from build123d import *

# Parameters (mm, degrees)
SKETCH1_R                         = 15.875
BOSS_EXTRUDE1_DEPTH               = 101.6
F_3_4_16_TAPPED_HOLE1_D           = 17.4625
F_3_4_16_TAPPED_HOLE1_DEPTH       = 42.926
F_3_4_16_TAPPED_HOLE1_CSINK_D     = 20.32
F_3_4_16_TAPPED_HOLE1_CSINK_ANGLE = 90
F_3_4_16_TAPPED_HOLE1_TIP         = 5.24626428


with BuildPart() as part:
    # Sketch1 → Boss-Extrude1 (new body)
    with BuildSketch(Plane(origin=(0, 0, 0), x_dir=(-1, 0, 0), z_dir=(0, 1, 0))):
        with Locations(Location((0, 0, 0), (0, 0, 90))):
            Circle(SKETCH1_R)
    extrude(amount=BOSS_EXTRUDE1_DEPTH)

    # Sketch2 → Cut-Revolve1 (revolve, cut)
    with BuildSketch(Plane(origin=(0, 0, 0), x_dir=(0, 1, 0), z_dir=(0, 0, 1)), mode=Mode.PRIVATE) as cut_revolve1_sk:
        Polygon((0, -6.35), (0, 0), (8.678122072, 0), (4.862657141, -6.35), align=None)
    revolve(cut_revolve1_sk.sketch.rotate(Axis((0, 0, 0), (0, 1, 0)), 90), axis=Axis((0, 0, 0), (0, 1, 0)), mode=Mode.SUBTRACT)

    # 3/4-16 Tapped Hole1
    with Locations(Plane(origin=(0, 101.6, 0), x_dir=(-1, 0, 0), z_dir=(0, 1, 0))):
        with Locations((0, 0)):
            CounterSinkHole(F_3_4_16_TAPPED_HOLE1_D / 2, F_3_4_16_TAPPED_HOLE1_CSINK_D / 2, depth=F_3_4_16_TAPPED_HOLE1_DEPTH, counter_sink_angle=F_3_4_16_TAPPED_HOLE1_CSINK_ANGLE)
            with Locations((0, 0, -(F_3_4_16_TAPPED_HOLE1_DEPTH + F_3_4_16_TAPPED_HOLE1_TIP / 2))):  # 118° drill point
                Cone(0, F_3_4_16_TAPPED_HOLE1_D / 2, F_3_4_16_TAPPED_HOLE1_TIP, mode=Mode.SUBTRACT)


solid = part.part
The listing builds one solid part. Answer for the finished solid, in the listing's coordinates (mm). A direction names the side the tool comes from. Coordinates: 2 decimals unless noted, no trailing zeros. Write each loop counter-clockwise with the first axis right and the second up, starting at its lowest first coordinate (ties: lowest second). Pieces come first, ordered by that corner, then holes. Notation, with made-up numbers: (89.25, 58) - (93.25, 58) arc R14 ccw to (93.25, 62) - close; hole circle Ø11 at (32, 25.25). An arc over 180 degrees is marked (long way). Return JSON: item names as keys, results as strings.
1. The part is cut by section C-C on x = -12. Determine the outline of the cut face in (y, z).
Final values:
{"outline": "(0, -10.39) - (101.6, -10.39) - (101.6, 10.39) - (0, 10.39) - close"}
2. Consider line 1 along X through (y, z) = (2.85, 0) (3 decimals); line 2 along X through (y, z) = (81, 0) (3 decimals); line 3 along Z through (x, y) = (14, 39). Determine where each line is inside the solid, lowest interval first.
Final values:
{"line 1": "-15.875 to -6.35, 6.35 to 15.875", "line 2": "-15.875 to -8.731, 8.731 to 15.875", "line 3": "-7.48 to 7.48"}
3. For a pull along X with two mould halves and no side action, classify faces 1 (the face through (-6.93, 79.13, -5.31)), 2 (the face through (-7, 0, 0)), 3 (the face through (-15.497, 50.089, -3.441)) as +X half, -X half, draft (parallel to the pull), parting line (faces both ways), or undercut.
Final values:
{"face 1": "undercut", "face 2": "draft", "face 3": "parting line"}
4. Which of the six approach directions +Z, -Z, +X, -X, +Y, -Y give full straight-line access (tool end or side, diameter ignored) to faces 4 (the face through (3.86, 2.4, 5.04)), 5 (the face through (-10.4, 101.6, -0.2))?
Final values:
{"face 4": "-Y", "face 5": "+Z, -Z, +X, -X, +Y"}
5. Each of these flat-tipped pins is pushed along its axis until it touches: pin 1 Ø14.5 at (x, z) = (0, 0) entering from -Y; pin 2 Ø2 at (x, y) = (7.5, 73) entering from +Z; pin 3 Ø4 at (x, y) = (11, 84.5) entering from -Z; pin 4 Ø3 at (x, z) = (0.5, -2.5) entering from -Y. Where does it stop, or does it pass through?
Final values:
{"pin 1": "y = 0", "pin 2": "z = 14.48", "pin 3": "z = -13.08", "pin 4": "y = 6.24"}
6. The part is cut by section D-D on x = 12.5. Determine the outline of the cut face in (y, z), then the cut area to 3 significant figures.
Final values:
{"outline": "(0, -9.79) - (101.6, -9.79) - (101.6, 9.79) - (0, 9.79) - close", "area": "1,990 mm^2"}
7. The part is cut by section B-B on y = 18.5. Determine the outline of the cut face in (x, z) (3 decimals).
Final values:
{"outline": "circle Ø31.75 at (0, 0)"}
